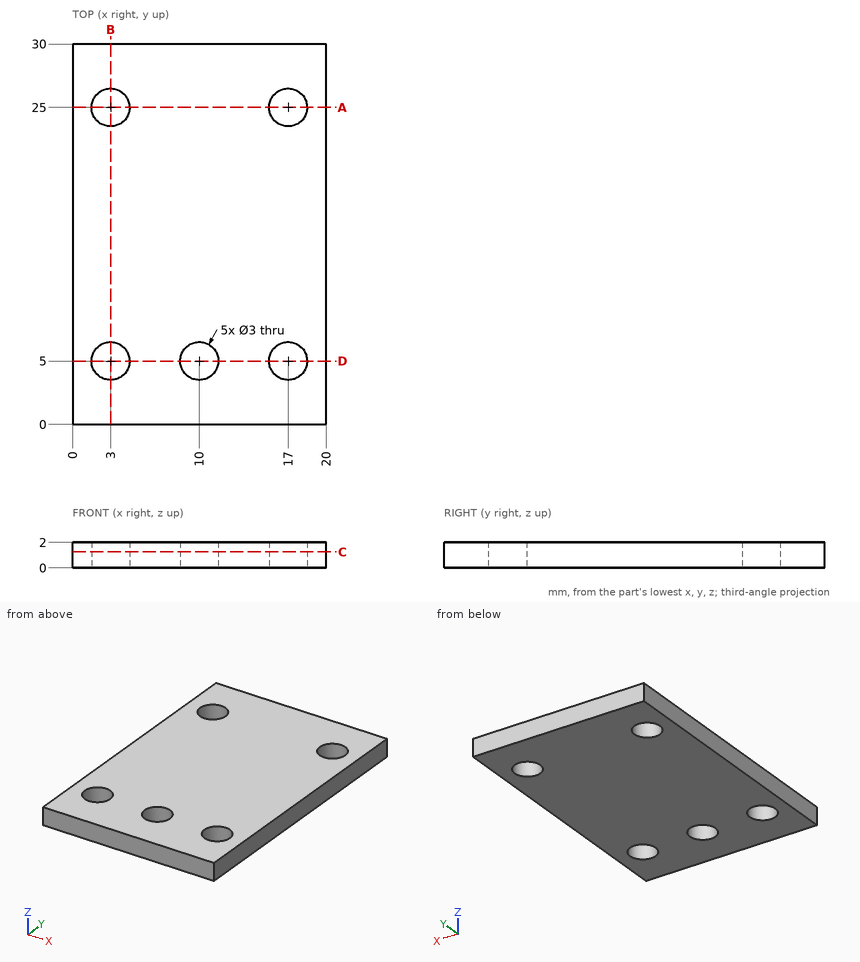
Here's the drawing with two shaded views (mm, measured from the low corner). I have some questions. Coordinates: 2 decimals unless noted, no trailing zeros. Order: outer loops, then holes, each group sorted by start corner. A loop starts at its lowest first (then second) coordinate and runs counter-clockwise, first axis right, second up.
Item 1: If we section it at D-D, the plane y = 5: List the corners of the cut face in (x, z) for me, then the cut area to 3 significant figures.
Response values:
outline: (0, 0) - (1.5, 0) - (1.5, 2) - (0, 2) - close; (4.5, 0) - (8.5, 0) - (8.5, 2) - (4.5, 2) - close; (11.5, 0) - (15.5, 0) - (15.5, 2) - (11.5, 2) - close; (18.5, 0) - (20, 0) - (20, 2) - (18.5, 2) - close
area: 22.0 mm2
Item 2: I'm going to push a flat-ended pin straight in: pin 1 Ø5 at (x, y) = (3, 25) entering from +Z. Where does the tip first touch, or does it pass through?
Response values:
pin 1: stops at z = 2
Item 3: If we section it at C-C, the plane z = 1.25: List the corners of the cut face in (x, y) for me.
Response values:
outline: (0, 0) - (20, 0) - (20, 30) - (0, 30) - close; hole circle Ø3 at (3, 5); hole circle Ø3 at (3, 25); hole circle Ø3 at (10, 5); hole circle Ø3 at (17, 5); hole circle Ø3 at (17, 25)
Item 4: If we section it at B-B, the plane x = 3: List the corners of the cut face in (y, z) for me.
Response values:
outline: (0, 0) - (3.5, 0) - (3.5, 2) - (0, 2) - close; (6.5, 0) - (23.5, 0) - (23.5, 2) - (6.5, 2) - close; (26.5, 0) - (30, 0) - (30, 2) - (26.5, 2) - close
Item 5: I need wall thicknesses on probe 1 along X at (y, z) = (5, 0.6); probe 2 along X at (y, z) = (25, 1.55); probe 3 along Y at (x, z) = (3, 0.75). Which ranges of each line are inside material? Lowest first, please.
Response values:
probe 1: x = 0 to 1.5, 4.5 to 8.5, 11.5 to 15.5, 18.5 to 20
probe 2: x = 0 to 1.5, 4.5 to 15.5, 18.5 to 20
probe 3: y = 0 to 3.5, 6.5 to 23.5, 26.5 to 30
Item 6: If we section it at A-A, the plane y = 25: List the corners of the cut face in (x, z) for me, then the cut area to 3 significant figures.
Response values:
outline: (0, 0) - (1.5, 0) - (1.5, 2) - (0, 2) - close; (4.5, 0) - (15.5, 0) - (15.5, 2) - (4.5, 2) - close; (18.5, 0) - (20, 0) - (20, 2) - (18.5, 2) - close
area: 28.0 mm2
